from build123d import *

# Parameters (mm, degrees)
SKETCH_1_W          = 30
SKETCH_1_H          = 30
EXTRUDE_1_DEPTH     = 120
SKETCH_2_W          = 9.747448714
SKETCH_2_H          = 5
SKETCH_2_W_2        = 5
SKETCH_2_H_2        = 9.747448714
CUT_EXTRUDE_1_DEPTH = 100
FILLET_1_R          = 8
CUT_EXTRUDE_2_DEPTH = 10


with BuildPart() as part:
    # 草图1 → 凸台-拉伸1 (new body)
    with BuildSketch(Plane(origin=(0, 0, 0), x_dir=(1, 0, 0), z_dir=(0, 1, 0))):
        Rectangle(SKETCH_1_W, SKETCH_1_H)
    extrude(amount=EXTRUDE_1_DEPTH)

    # 草图2 → 切除-拉伸1 (cut)
    with BuildSketch(Plane(origin=(0, 120, 0), x_dir=(1, 0, 0), z_dir=(0, 1, 0))):
        with Locations((-7.373724357, 0)):
            Rectangle(SKETCH_2_W, SKETCH_2_H)
        Rectangle(SKETCH_2_W_2, SKETCH_2_H)
        with Locations((0, -7.373724357)):
            Rectangle(SKETCH_2_W_2, SKETCH_2_H_2)
        with Locations((7.373724357, 0)):
            Rectangle(SKETCH_2_W, SKETCH_2_H)
        with Locations((0, 7.373724357)):
            Rectangle(SKETCH_2_W_2, SKETCH_2_H_2)
        with BuildLine():
            ThreePointArc((-12.247448714, 2.5), (-12.5, 0), (-12.247448714, -2.5))
            Line((-12.247448714, -2.5), (-12.247448714, 2.5))
        make_face()
        with BuildLine():
            ThreePointArc((2.5, 12.247448714), (0, 12.5), (-2.5, 12.247448714))
            Line((-2.5, 12.247448714), (2.5, 12.247448714))
        make_face()
        with BuildLine():
            Line((12.247448714, 2.5), (12.247448714, -2.5))
            ThreePointArc((12.247448714, -2.5), (12.436701913, -1.256362025), (12.5, 0))
            ThreePointArc((12.5, 0), (12.436701913, 1.256362025), (12.247448714, 2.5))
        make_face()
        with BuildLine():
            Line((2.5, -12.247448714), (-2.5, -12.247448714))
            ThreePointArc((-2.5, -12.247448714), (0, -12.5), (2.5, -12.247448714))
        make_face()
    extrude(amount=-CUT_EXTRUDE_1_DEPTH, mode=Mode.SUBTRACT)

    # 圆角1
    fillet_1_edges = [part.edges().sort_by_distance(p)[0] for p in [
        (-2.5, 70, -2.5),
        (2.5, 70, -2.5),
        (2.5, 70, 2.5),
        (-2.5, 70, 2.5),
    ]]
    fillet(fillet_1_edges, radius=FILLET_1_R)

    # 草图4 → 切除-拉伸2 (cut)
    with BuildSketch(Plane(origin=(0, 120, 0), x_dir=(1, 0, 0), z_dir=(0, 1, 0))):
        Polygon((4.254858786, -9.911713035), (9.911713035, -4.254858786), (13.447246941, -7.790392692), (7.790392692, -13.447246941), align=None)
    extrude(amount=-CUT_EXTRUDE_2_DEPTH, mode=Mode.SUBTRACT)


solid = part.part
Input: part model. Units: mm. Frame: model coordinates. A direction names the side the tool comes from. Coordinates: 2 decimals unless noted, no trailing zeros. Loops run counter-clockwise (first coordinate to the right, second up) from the corner with the lowest first, then second, coordinate; pieces in that order, holes last.
Q1. Cut plane C-C (x = -0.25). Output: boundary loops of the cut face in (y, z), then the cut area to 3 significant figures.
Q2. Draft query along Z for faces 3 (the face through (11.655, 115.07, 5.998)), 4 (the face through (15, 59, 0)), 5 (the face through (0, 59, -15)). Return one class per face: +Z half, -Z half, draft (parallel to the pull), parting line (faces both ways), or undercut.
Q3. Cut plane A-A (y = 73). Output: boundary loops of the cut face in (x, z).
Q4. Cut plane D-D (x = 6.25). Output: boundary loops of the cut face in (y, z).
Q5. Set-up query: faces 1 (the face through (-4, 120, -7)), 2 (the face through (4.781, 69.3, 4.906)). Return all of +Z, -Z, +X, -X, +Y, -Y with unobstructed straight access to the full face (end or side cutting, diameter ignored); none if empty.
Q6. Material intervals for line 1 (Z direction, x = -11.5, y = 67); line 2 (Y direction, x = 3.5, z = -3.25); line 3 (X direction, y = 97, z = 7.75), sorted ascending.
Q7. Contact query for a flat-ended pin moving along its axis: pin 1 (4.5 mm diameter, centred on x = 9.5, z = 8.5, fed in from +Y). Output: stop coordinate, or through.
Q8. Cut plane B-B (z = -4.5). Output: boundary loops of the cut face in (x, y).
Working result:
1. outline: (0, -15) - (120, -15) - (120, -12.5) - (20, -12.5) - (20, 12.5) - (120, 12.5) - (120, 15) - (0, 15) - close
1. area: 1,100 mm2
2. face 3: undercut
2. face 4: draft
2. face 5: -Z half
3. outline: (-15, -15) - (15, -15) - (15, 15) - (-15, 15) - close; hole (-12.25, -2.5) - (-10.5, -2.5) arc R8 cw to (-2.5, -10.5) - (-2.5, -12.25) arc R12.5 ccw to (2.5, -12.25) - (2.5, -10.5) arc R8 cw to (10.5, -2.5) - (12.25, -2.5) arc R12.5 ccw to (12.25, 2.5) - (10.5, 2.5) arc R8 cw to (2.5, 10.5) - (2.5, 12.25) arc R12.5 ccw to (-2.5, 12.25) - (-2.5, 10.5) arc R8 cw to (-10.5, 2.5) - (-12.25, 2.5) arc R12.5 ccw to start
4. outline: (0, -15) - (120, -15) - (120, -3.72) - (20, -3.72) - (20, 3.72) - (120, 3.72) - (120, 7.92) - (110, 7.92) - (110, 11.91) - (120, 11.91) - (120, 15) - (0, 15) - close
5. face 1: +Z, -Z, +X, -X, +Y
5. face 2: +Y
6. line 1: z = -15 to -2.5, 2.5 to 15
6. line 2: y = 0 to 20
6. line 3: x = -15 to -2.99, 2.99 to 15
7. pin 1: stops at y = 110
8. outline: (-15, 0) - (15, 0) - (15, 120) - (5.21, 120) - (5.21, 20) - (-5.21, 20) - (-5.21, 120) - (-15, 120) - close
